Autodesk Inventor part; units mm, degrees
ref_plane "IDS_WORKPLANE{1}" through (-6.35, 0, 0) normal (1, 0, 0) x (0, 0, -1)
ref_plane "Work Plane2" through (-3.175, 0, 0) normal (0, 0, -1) x (1, 0, 0)
ref_plane "YZ Plane" through (0, 0, 0) normal (1, 0, 0) x (0, 1, 0)
sketch "Sketch1" plane through (0, 0, 0) normal (0, 0, 1) x (1, 0, 0)
  line L0 (-6.35, 0) -> (38.1, 0)
  line L1 (38.1, 0) -> (38.1, 3.175)
  line L2 (38.1, 3.175) -> (0, 3.175)
  line L3 (0, 3.175) -> (0, 4.7625)
  line L4 (-17.3035, 0) -> (47.3339, 0)
  line L5 (0, -0.9525) -> (0, 5.715)
  line L6 (0, 4.7625) -> (-6.35, 4.7625)
  line L7 (-6.35, 0) -> (-6.35, 4.7625)
  arc A0 (-2.5645, 0) -> (-3.302, 2.7526) centre (-8.0696, 0) ccw
  line L8 (-6.35, 2.7526) -> (-3.302, 2.7526)
  line L9 (12.7, 3.175) -> (0, 3.175) construction
  dimension "d0" = 38.1
  dimension "d1" = 6.35
  dimension "d2" = 6.35
  dimension "d5" = 9.525
  dimension "d13" = 5.5051
  dimension "d14" = 5.5051
  dimension "d15" = 3.048
revolve "Body" add sketch "Sketch1" angle 360 about axis through (-6.35, 0, 0) along (1, 0, 0) contours A0 L8 L7 L6 L3 L5 L0 | L5 L2 L1 L0
ref_plane "IDS_WORKPLANE{1}" through (-6.35, 0, 0) normal (1, 0, 0) x (0, 0, -1)
sketch "Sketch2" plane through (-6.35, 0, 0) normal (1, 0, 0) x (0, 0, -1)
  line L0 (0, -6.6675) -> (0, 6.6675)
  line L1 (6.6675, 0) -> (-6.6675, 0)
  circle A0 centre (0, 0) radius 4.7625
  line L2 (2.6768, 0.6414) -> (2.2959, 0.6414)
  line L3 (0, 0) -> (2.6768, 0.6414) construction
  line L4 (0, 0) -> (4.0727, 3.8613) construction
  line L5 (0, 0) -> (0.783, 2.6389) construction
  line L6 (0, 0) -> (1.3763, 2.3838) construction
  line L7 (0.783, 2.6389) -> (0.5925, 2.309)
  line L8 (1.8938, 1.9975) -> (1.7034, 1.6676)
  line L9 (0, 0) -> (1.8938, 1.9975) construction
  arc A1 (2.3838, 0) -> (2.2959, 0.6414) centre (0, 0) ccw
  arc A2 (1.7034, 1.6676) -> (0.5925, 2.309) centre (0, 0) ccw
  arc A3 (2.7526, 0) -> (2.6768, 0.6414) centre (0, 0) ccw
  arc A4 (1.8938, 1.9975) -> (0.783, 2.6389) centre (0, 0) ccw
  arc A5 (2.6768, 0.6414) -> (1.6232, 2.223) centre (0, 0) ccw construction
  arc A6 (2.2959, 0.6414) -> (1.7034, 1.6676) centre (0, 0) ccw construction
  line L10 (2.6768, -0.6414) -> (2.2959, -0.6414)
  line L11 (0.783, -2.6389) -> (0.5925, -2.309)
  line L12 (1.8938, -1.9975) -> (1.7034, -1.6676)
  arc A7 (2.2959, -0.6414) -> (2.3838, 0) centre (0, 0) ccw
  arc A8 (0.5925, -2.309) -> (1.7034, -1.6676) centre (0, 0) ccw
  arc A9 (2.6768, -0.6414) -> (2.7526, 0) centre (0, 0) ccw
  arc A10 (0.783, -2.6389) -> (1.8938, -1.9975) centre (0, 0) ccw
  line L13 (-2.6768, 0.6414) -> (-2.2959, 0.6414)
  line L14 (-0.783, 2.6389) -> (-0.5925, 2.309)
  line L15 (-1.8938, 1.9975) -> (-1.7034, 1.6676)
  arc A11 (-2.2959, 0.6414) -> (-2.3838, 0) centre (0, 0) ccw
  arc A12 (-0.5925, 2.309) -> (-1.7034, 1.6676) centre (0, 0) ccw
  arc A13 (-2.6768, 0.6414) -> (-2.7526, 0) centre (0, 0) ccw
  arc A14 (-0.783, 2.6389) -> (-1.8938, 1.9975) centre (0, 0) ccw
  line L16 (-0.783, -2.6389) -> (-0.5925, -2.309)
  arc A15 (-1.7034, -1.6676) -> (-0.5925, -2.309) centre (0, 0) ccw
  line L17 (-1.8938, -1.9975) -> (-1.7034, -1.6676)
  arc A16 (-1.8938, -1.9975) -> (-0.783, -2.6389) centre (0, 0) ccw
  arc A17 (-2.3838, 0) -> (-2.2959, -0.6414) centre (0, 0) ccw
  line L18 (-2.6768, -0.6414) -> (-2.2959, -0.6414)
  arc A18 (-2.7526, 0) -> (-2.6768, -0.6414) centre (0, 0) ccw
  point P0 (1.3763, -2.3838)
  point P1 (-1.3763, 2.3838)
  point P2 (-1.3763, -2.3838)
  dimension "d19" = 0.6413
  dimension "d20" = 1.2827
  dimension "d21" = 33.052
  dimension "d22" = 5.5051
  dimension "d23" = 4.7676
extrude "Slot" add sketch "Sketch2" along normal up to next contours A1 L2 A3 L1 | L1 A9 L10 A7 | A17 L18 A18 L1 | L1 A13 L13 A11 | A4 L8 A2 L7 | L11 A8 L12 A10 | L14 A12 L15 A14 | A16 L17 A15 L16
fillet "Fillet1" radius 0.635 1 edges at (-6.35, -4.7625, 0)
thread "Thread"
chamfer "Chamfer1" distance 0.541 distance2 0.541 1 edges at (38.1, -3.175, 0) measured on face at (38.1, -0.6107, -1.4381)
ref_plane "Work Plane2" through (-3.175, 0, 0) normal (0, 0, -1) x (1, 0, 0)
equation "\"d19\" = 0.5 * SBR"
equation "\"d20\" = SBR"
equation "\"d22\" = 1.1547 * SW"
equation "\"d23\" = SW"
equation "\"d17\" = INTI"
equation "\"d24\" = RR"
equation "\"d6\" = GEL"
equation "\"d9\" = -0.5 * SPD + 0.5 * NND"
equation "\"d10\" = GUL"
equation "\"d0\" = NLG"
equation "\"d1\" = KOH"
equation "\"d2\" = NND"
equation "\"d5\" = KOD"
equation "\"d13\" = 1.1547 * SW"
equation "\"d14\" = 1.1547 * SW"
equation "\"d15\" = INTI"
equation "\"NND\" = 6.35"
equation "\"NLG\" = 38.1"
equation "\"GEL\" = 25.4"
equation "\"KOD\" = 9.525"
equation "\"KOH\" = 6.35"
equation "\"SPD\" = GD1"
equation "\"GUL\" = 0.54102"
equation "\"SBR\" = 1.2827"
equation "\"INTI\" = 3.048"
equation "\"d11\" = -KOH"
equation "\"SW\" = 4.76758"
equation "\"d16\" = 1.1547 * SW"
equation "\"d18\" = SW"
equation "\"RR\" = 0.635"
equation "\"TOA\" = 30deg"
equation "\"GD1\" = 5.26796"
equation "\"THREADDIA\" = 6.35"
equation "\"BDM\" = NND"
equation "\"GD\" = NND"
equation "\"GAL\" = 1.36068"
equation "\"E0\" = 5.55498"
properties part number "ANSI B18.3 - 1/4-28 UNF - 1.5" material "Steel, Mild"
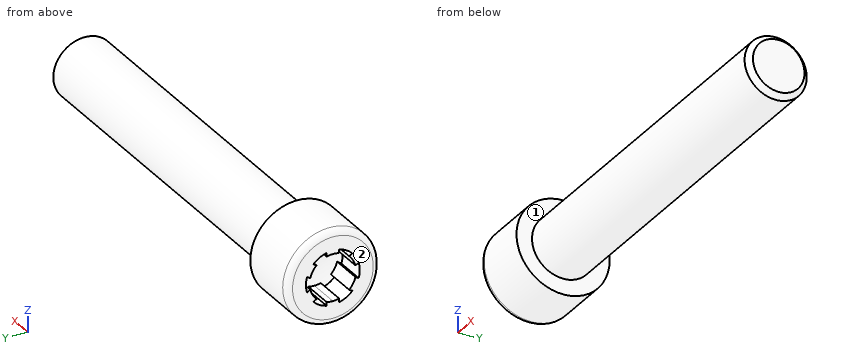
Can you work these out from the model? Positions are in its coordinate system, mm. Face numbers are marked on the shaded views. A direction names the side the tool comes from. Coordinates: 2 decimals unless noted, no trailing zeros. Order: outer loops, then holes, each group sorted by start corner. A loop starts at its lowest first (then second) coordinate and runs counter-clockwise, first axis right, second up.
1. For the marked faces 1 and 2, which set-ups out of +Z, -Z, +X, -X, +Y, -Y let a thin tool reach every point of the face, with its end or its side?
2. I need wall thicknesses on line 1 (X direction, y = -0.75, z = -3.25); line 2 (Z direction, x = 28, y = 0) (3 decimals); line 3 (Y direction, x = 22, z = 0.25). Which ranges of each line are inside material? Lowest first, please.
3. I'm going to push flat-ended pins straight in: pin 1 (4 mm diameter, centred on x = 3.5, y = 3, fed in from +Z); pin 2 (1 mm diameter, centred on y = 3, z = -4, fed in from +X); pin 3 (1 mm diameter, centred on x = 32, y = -1, fed in from -Z). Where does each tip first touch, or does it pass through?
4. If we section it at A-A (x = 25): Please give me the cut outline in (y, z) (3 decimals).
Entries:
1. face 1: +X
1. face 2: +Z, -Z, -X, +Y, -Y
2. line 1: x = -6.35 to 0
2. line 2: z = -3.175 to 3.175
2. line 3: y = -3.17 to 3.17
3. pin 1: stops at z = 3.01
3. pin 2: stops at x = 0
3. pin 3: stops at z = -3.14
4. outline: circle Ø6.35 at (0, 0)
